Build history of the part. All positions in model axes, mm. A direction names the side the tool comes from. Coordinates: 2 decimals unless noted, no trailing zeros. Loops run counter-clockwise (first coordinate to the right, second up) from the corner with the lowest first, then second, coordinate; pieces in that order, holes last. Notation, with made-up numbers: (22, 0) - (52, 0) arc R12 ccw to (52, 15) - close; hole circle Ø6 at (65, 66). An arc over 180 degrees is marked (long way). One line per item, written item: value.
```python
from build123d import *

# Parameters (mm, degrees)
BOSS_EXTRUDE1_DEPTH = 110
SKETCH2_R           = 1.75
CUT_EXTRUDE1_DEPTH  = 111.905365064
CUT_EXTRUDE2_DEPTH  = 112.360899781
FILLET1_R           = 4
FILLET2_R           = 1


with BuildPart() as part:
    # Sketch1 → Boss-Extrude1 (new, symmetric)
    with BuildSketch(Plane(origin=(0, 0, 0), x_dir=(0, 0, -1), z_dir=(1, 0, 0))):
        Polygon((-13, -1.5), (-13, 1.5), (-3, 1.5), (-3, 10), (0, 10), (0, -10), (-3, -10), (-3, -1.5), align=None)
    extrude(amount=BOSS_EXTRUDE1_DEPTH, both=True)

    # Sketch2 → Cut-Extrude1 (cut, through all)
    with BuildSketch(Plane.XY.offset(3)):
        with Locations((-15, -5.75)):
            Circle(SKETCH2_R)
        with Locations((-45, -5.75)):
            Circle(SKETCH2_R)
        with Locations((-75, -5.75)):
            Circle(SKETCH2_R)
        with Locations((-105, -5.75)):
            Circle(SKETCH2_R)
        with Locations(Location((105, -5.75, 0), (0, 0, 180))):
            Circle(SKETCH2_R)
        with Locations(Location((75, -5.75, 0), (0, 0, 180))):
            Circle(SKETCH2_R)
        with Locations(Location((45, -5.75, 0), (0, 0, 180))):
            Circle(SKETCH2_R)
        with Locations(Location((15, -5.75, 0), (0, 0, 180))):
            Circle(SKETCH2_R)
        with Locations((15, 5.75)):
            Circle(SKETCH2_R)
        with Locations((45, 5.75)):
            Circle(SKETCH2_R)
        with Locations((75, 5.75)):
            Circle(SKETCH2_R)
        with Locations((105, 5.75)):
            Circle(SKETCH2_R)
        with Locations(Location((-105, 5.75, 0), (0, 0, 180))):
            Circle(SKETCH2_R)
        with Locations(Location((-75, 5.75, 0), (0, 0, 180))):
            Circle(SKETCH2_R)
        with Locations(Location((-45, 5.75, 0), (0, 0, 180))):
            Circle(SKETCH2_R)
        with Locations(Location((-15, 5.75, 0), (0, 0, 180))):
            Circle(SKETCH2_R)
    extrude(amount=-CUT_EXTRUDE1_DEPTH, mode=Mode.SUBTRACT)

    # Sketch3 → Cut-Extrude2 (cut, through all)
    with BuildSketch(Plane(origin=(0, 1.5, 0), x_dir=(1, 0, 0), z_dir=(0, 1, 0))):
        with BuildLine():
            Line((50, -13), (110, -13))
            Line((110, -13), (110, -6))
            Line((110, -6), (51.525650044, -12.910166224))
            ThreePointArc((51.525650044, -12.910166224), (50.764146283, -12.977522123), (50, -13))
        make_face()
        with BuildLine():
            Line((-51.525650044, -12.910166224), (-110, -6))
            Line((-110, -6), (-110, -13))
            Line((-110, -13), (-50, -13))
            ThreePointArc((-50, -13), (-50.764146283, -12.977522123), (-51.525650044, -12.910166224))
        make_face()
    extrude(amount=-CUT_EXTRUDE2_DEPTH, mode=Mode.SUBTRACT)

    # Fillet1
    fillet1_edges = [part.edges().sort_by_distance(p)[0] for p in [
        (110, -10, 1.5),
        (110, 10, 1.5),
        (-110, 10, 1.5),
        (-110, -10, 1.5),
    ]]
    fillet(fillet1_edges, radius=FILLET1_R)

    # Fillet2
    fillet2_edges = [part.edges().sort_by_distance(p)[0] for p in [
        (0, -1.5, 3),
        (0, 1.5, 3),
    ]]
    fillet(fillet2_edges, radius=FILLET2_R)


solid = part.part
```
Item 1: Pull direction Y, two halves, no side cores. Call faces 1 (the face through (-110, 0, 2)), 2 (the face through (-15.81, 7.3, 1.52)), 3 (the face through (2, -1.5, 7)): released by +Y, released by -Y, zero draft, split by the parting line, or undercut.
Check result:
face 1: zero draft
face 2: undercut
face 3: released by -Y
Item 2: Cut at C-C, the plane x = 86. Write the cut outline in (y, z), then the cut area to 3 significant figures.
Check result:
outline: (-10, 0) - (10, 0) - (10, 3) - (2.5, 3) arc R1 cw to (1.5, 4) - (1.5, 8.84) - (-1.5, 8.84) - (-1.5, 4) arc R1 cw to (-2.5, 3) - (-10, 3) - close
area: 77.9 mm^2
Item 3: Tool access for faces 4 (the face through (46.617, 5.08, 1.521)), 5 (the face through (2, -6, 3)): list every direction of +Z, -Z, +X, -X, +Y, -Y with a clear straight run to the whole face (end or side of a thin tool).
Check result:
face 4: +Z, -Z
face 5: +Z, +X, -X, -Y
Item 4: Cut at B-B, the plane z = 9.75. Write the cut outline in (x, y).
Check result:
outline: (-78.27, -1.5) - (78.27, -1.5) - (78.27, 1.5) - (-78.27, 1.5) - close
Item 5: Cut at A-A, the plane x = -4. Write the cut outline in (y, z).
Check result:
outline: (-10, 0) - (10, 0) - (10, 3) - (2.5, 3) arc R1 cw to (1.5, 4) - (1.5, 13) - (-1.5, 13) - (-1.5, 4) arc R1 cw to (-2.5, 3) - (-10, 3) - close
Item 6: Drop flat-ended pins along their axis: P1, Ø5.5, axis at x = -15, y = 5.75, coming from the -Z side; P2, Ø4, axis at x = 15, y = 5.75, coming from the +Z side; P3, Ø7, axis at x = -39.5, z = 9.5, coming from the +Y side. Give the stop position or say it passes through.
Check result:
P1: stops at z = 0
P2: stops at z = 3
P3: stops at y = 1.5
Item 7: Probe probe 1 along Y at (x, z) = (-75, 1.25); probe 2 along Z at (x, y) = (60, -4.5); probe 3 along Y at (x, z) = (-80.5, 4). List the from-to ranges inside material, lowest first. Write a range as from..to.
Check result:
probe 1: y = -10..-7.5, -4..4, 7.5..10
probe 2: z = 0..3
probe 3: y = -1.5..1.5
